```python
from build123d import *

# Parameters (mm, degrees)
ESQUISSE1_W             = 176
ESQUISSE1_H             = 106
BOSS_EXTRU_1_DEPTH      = 3
CONG_1_R                = 3
ESQUISSE3_R             = 6
ENL_V_MAT_EXTRU_2_DEPTH = 10
ESQUISSE4_W             = 15.3
ESQUISSE4_H             = 15.3
ENL_V_MAT_EXTRU_3_DEPTH = 10


with BuildPart() as part:
    # Esquisse1 → Boss.-Extru.1 (new body)
    with BuildSketch(Plane(origin=(0, 0, 0), x_dir=(1, 0, 0), z_dir=(0, 1, 0))):
        Rectangle(ESQUISSE1_W, ESQUISSE1_H)
    extrude(amount=BOSS_EXTRU_1_DEPTH)

    # Congé1
    cong_1_edges = [part.edges().sort_by_distance(p)[0] for p in [
        (88, 1.5, 53),
        (-88, 1.5, 53),
        (-88, 1.5, -53),
        (88, 1.5, -53),
    ]]
    fillet(cong_1_edges, radius=CONG_1_R)

    # Esquisse3 → Enlèv. mat.-Extru.2 (cut)
    with BuildSketch(Plane.XZ):
        with Locations((78, 14)):
            Circle(ESQUISSE3_R)
    extrude(amount=-ENL_V_MAT_EXTRU_2_DEPTH, mode=Mode.SUBTRACT)

    # Esquisse4 → Enlèv. mat.-Extru.3 (cut)
    with BuildSketch(Plane.XZ):
        with Locations((-71.961639113, -36.263401643)):
            Rectangle(ESQUISSE4_W, ESQUISSE4_H)
    extrude(amount=-ENL_V_MAT_EXTRU_3_DEPTH, mode=Mode.SUBTRACT)


solid = part.part
```
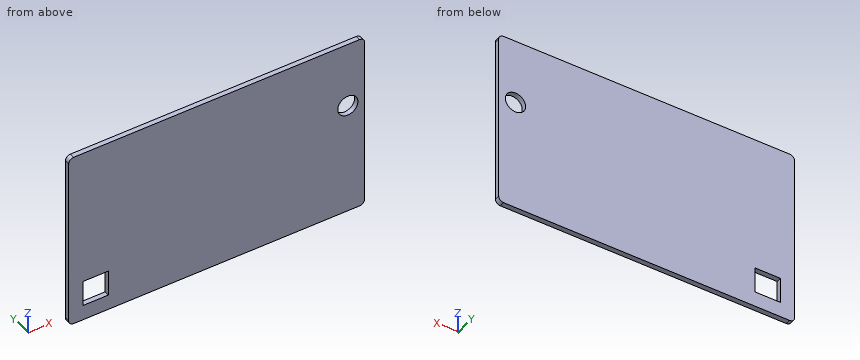
Build history of the part. All positions in model axes, mm. Round coordinates to 2 decimals unless told otherwise and drop trailing zeros. Order: outer loops, then holes, each group sorted by start corner. A loop starts at its lowest first (then second) coordinate and runs counter-clockwise, first axis right, second up. Notation, with made-up numbers: (-36.75, 19) -> (-16.75, 19) arc R12 ccw to (-16.75, 34) -> close; hole circle Ø2 at (-24, 76). An arc over 180 degrees is marked (long way). Answer in a Markdown table with one row per item.
1) Wall check: L1, parallel to X at y = 2.2, z = -41; L2, parallel to Z at x = 78, y = 1.35. Give the ranges that are in metal, low to high.
Values:
| item | result |
|---|---|
| L1 | -88 to -79.61, -64.31 to 88 |
| L2 | -53 to 8, 20 to 53 |
2) Band-saw the part on B-B on z = 14. Give the cut face in (x, y), and give its area (3 significant figures).
Values:
| item | result |
|---|---|
| outline | (-88, 0) -> (72, 0) -> (72, 3) -> (-88, 3) -> close; (84, 0) -> (88, 0) -> (88, 3) -> (84, 3) -> close |
| area | 492 mm2 |
3) Band-saw the part on C-C on y = 1.9. Give the cut face in (x, z).
Values:
| item | result |
|---|---|
| outline | (-88, -50) arc R3 ccw to (-85, -53) -> (85, -53) arc R3 ccw to (88, -50) -> (88, 50) arc R3 ccw to (85, 53) -> (-85, 53) arc R3 ccw to (-88, 50) -> close; hole (-79.61, -43.91) -> (-64.31, -43.91) -> (-64.31, -28.61) -> (-79.61, -28.61) -> close; hole circle Ø12 at (78, 14) |
4) Band-saw the part on A-A on x = -75. Give the cut face in (y, z), and give its area (3 significant figures).
Values:
| item | result |
|---|---|
| outline | (0, -53) -> (3, -53) -> (3, -43.91) -> (0, -43.91) -> close; (0, -28.61) -> (3, -28.61) -> (3, 53) -> (0, 53) -> close |
| area | 272 mm2 |
